```python
from build123d import *

# Parameters (mm, degrees)
F0_R     = 10
F0_R_2   = 5
F1_DEPTH = 25
F2_DEPTH = 25
F3_R     = 4.99999


# Not quite as in the source:
# - a fillet or chamfer is up to 0.001 mm smaller than in the source, because OpenCascade refuses the exact size


with BuildPart() as f1:
    # F0 (on Top) → F1 (new body)
    with BuildSketch(Plane.XY):
        Circle(F0_R)
        Circle(F0_R_2, mode=Mode.SUBTRACT)
    extrude(amount=F1_DEPTH)

    # F0 (on Top) → F2 (join)
    with BuildSketch(Plane.XY):
        Circle(F0_R)
        Circle(F0_R_2, mode=Mode.SUBTRACT)
    extrude(amount=F2_DEPTH)

    # F3 (radius 5 in the source; OpenCascade refuses exactly that, so slightly less here)
    f3_edges = [f1.edges().sort_by_distance(p)[0] for p in [
        (-10, 0, 25),
    ]]
    fillet(f3_edges, radius=F3_R)


solid = f1.part
```
CAD build for the part. Positions are in the model's coordinates, mm. Coordinates: 2 decimals unless noted, no trailing zeros. Loops run counter-clockwise (first coordinate to the right, second up) from the corner with the lowest first, then second, coordinate; pieces in that order, holes last. Notation, with made-up numbers: (56.25, -32) - (88.25, -32) arc R21 ccw to (88.25, -23) - close; hole circle Ø10 at (-20, 41.25). An arc over 180 degrees is marked (long way). Use CSV: the item, a comma, the result in double quotes. Start each with the question number.
Q1. Cut at C-C, the plane z = 7.5. List the corners of the cut face in (x, y), then the cut area to 3 significant figures.
Q2. Cut at D-D, the plane z = 23.75. List the corners of the cut face in (x, y), then the cut area to 3 significant figures.
Q3. Two-plate mould, pull along X, no slides. Class faces 1 (the cylindrical face through (-1.08, -4.88, 12.32)), 2 (the flat face through (-5, -2, 0)), 3 (the cylindrical face through (-2.17, -9.76, 9.86)): +X half, -X half, draft (parallel to the pull), parting line (faces both ways), or undercut.
Q4. Drop flat-ended pins along their axis: P1, Ø6, axis at y = -1.5, z = 12, coming from the +X side; P2, Ø2, axis at x = 7, z = 10, coming from the -Y side; P3, Ø6, axis at y = -4, z = 7, coming from the +X side; P4, Ø2, axis at y = 5.5, z = 5, coming from the +X side. Give the stop position or say it passes through.
Q5. Probe probe 1 along Y at (x, z) = (0, 19.25); probe 2 along X at (y, z) = (-2, 12.5); probe 3 along Y at (x, z) = (-4.25, 15.25). List the from-to ranges inside material, lowest first. Write a range as from..to.
Here are the results:
1,outline,"circle Ø20 at (0, 0); hole circle Ø10 at (0, 0)"
1,area,"236 mm2"
2,outline,"circle Ø16.61 at (0, 0); hole circle Ø10 at (0, 0)"
2,area,"138 mm2"
3,face 1,"undercut"
3,face 2,"draft"
3,face 3,"parting line"
4,P1,"x = 10"
4,P2,"y = -8"
4,P3,"x = 9.95"
4,P4,"x = 8.93"
5,probe 1,"-10..-5, 5..10"
5,probe 2,"-9.8..-4.58, 4.58..9.8"
5,probe 3,"-9.05..-2.63, 2.63..9.05"
